```python
from build123d import *
from build123d.topology import SkipClean

# Parameters (mm, degrees)
BOSS_EXTRUDE1_DEPTH                  = 15
SKETCH2_R                            = 12.5
BOSS_EXTRUDE2_DEPTH                  = 22
BOSS_EXTRUDE2_DIRECTION_2_REACH      = 23.768
BOSS_EXTRUDE2_DIRECTION_2_END_RADIUS = 40.5
SKETCH3_R                            = 9.9
BOSS_EXTRUDE3_DEPTH                  = 13
CHAMFER1_SIZE                        = 1
FILLET7_R                            = 3


with BuildPart() as part:
    # Sketch1 → Boss-Extrude1 (new, symmetric)
    with BuildSketch(Plane(origin=(0, 0, 0), x_dir=(1, 0, 0), z_dir=(0, 1, 0))):
        with BuildLine():
            ThreePointArc((2.261526721, 12.825755375), (0, 0), (2.261526721, -12.825755375))
            ThreePointArc((2.261526721, -12.825755375), (1.365018004, -14.748324521), (-0.557551142, -13.851815805))
            ThreePointArc((-0.557551142, -13.851815805), (-3, 0), (-0.557551142, 13.851815805))
            ThreePointArc((-0.557551142, 13.851815805), (1.365018004, 14.748324521), (2.261526721, 12.825755375))
        make_face()
    extrude(amount=BOSS_EXTRUDE1_DEPTH, both=True)

    # Sketch2 → Boss-Extrude2 (add)
    with BuildSketch(Plane.ZY.offset(3)):
        with Locations(Location((0, 0, 0), (0, 0, 180))):
            Circle(SKETCH2_R)
    extrude(amount=BOSS_EXTRUDE2_DEPTH)

    # Boss-Extrude2 direction 2: up to this cylinder (the profile starts outside it)
    with SkipClean():  # the faces are left unmerged after this step: merging them gives an invalid solid
        boss_extrude2_direction_2_end = Plane(origin=(37.5, 0, 0), z_dir=(0, -1, 0)) * Cylinder(BOSS_EXTRUDE2_DIRECTION_2_END_RADIUS, 129.536, mode=Mode.PRIVATE)
        # Sketch2 → Boss-Extrude2 direction 2 (add, up to the surface)
        with BuildSketch(Plane.ZY.offset(3), mode=Mode.PRIVATE) as boss_extrude2_direction_2_sk1:
            with Locations(Location((0, 0, 0), (0, 0, 180))):
                Circle(SKETCH2_R)
        boss_extrude2_direction_2_tool1 = extrude(boss_extrude2_direction_2_sk1.sketch, amount=-BOSS_EXTRUDE2_DIRECTION_2_REACH, mode=Mode.PRIVATE) - boss_extrude2_direction_2_end
        add(boss_extrude2_direction_2_tool1.solids().sort_by_distance((-3, 0, 0))[0])
        add(boss_extrude2_direction_2_tool1.solids().sort_by_distance((-3, 0, 0))[1])

    # Sketch3 → Boss-Extrude3 (add)
    with BuildSketch(Plane.ZY.offset(25)):
        with Locations(Location((0, 0, 0), (0, 0, 180))):
            Circle(SKETCH3_R)
    extrude(amount=BOSS_EXTRUDE3_DEPTH)

    # Chamfer1
    chamfer1_edges = [part.edges().sort_by_distance(p)[0] for p in [
        (-38, 0, 9.9),
    ]]
    chamfer(chamfer1_edges, length=CHAMFER1_SIZE)

    # Fillet7
    fillet7_edges = [part.edges().sort_by_distance(p)[0] for p in [
        (-1.022720569, 0, 12.5),
    ]]
    fillet(fillet7_edges, radius=FILLET7_R)


solid = part.part
```
The model under review builds one solid part; all positions refer to its coordinate system, in mm. A direction names the side the tool comes from. Round coordinates to 2 decimals unless told otherwise and drop trailing zeros. Write each loop counter-clockwise with the first axis right and the second up, starting at its lowest first coordinate (ties: lowest second). Pieces come first, ordered by that corner, then holes. Notation, with made-up numbers: (41.5, 65) - (69.5, 65) arc R18 ccw to (69.5, 86) - close; hole circle Ø7 at (30.5, 27). An arc over 180 degrees is marked (long way). One line per question, with ' | ' between items.
Item 1: For faces 4 (the face through (-1.46, -12.41, -11.06)), 5 (the face through (-1.34, -12.02, 11.48)), 6 (the face through (-1.46, 12.46, -11.06)), 7 (the face through (-13.868, -3.755, -11.923)), 8 (the face through (-0.3, -15, -0.2)), list the 3-axis set-ups (+Z, -Z, +X, -X, +Y, -Y) from which the entire face can be reached by the end or side of a thin tool; tool diameter is ignored.
Resolved:
face 4: -Z, -X, -Y | face 5: +Z, -X, -Y | face 6: -Z, -X, +Y | face 7: -X | face 8: +Z, -Z, +X, -X, -Y
Item 2: Add section A-A, the plane x = -9. Give the boundary of the cut face in (y, z), then the cut area to 3 significant figures.
Resolved:
outline: circle Ø25 at (0, 0) | area: 491 mm2
Item 3: To check wall thickness, follow probe 1 along X at (y, z) = (8, 0.25); probe 2 along Y at (x, z) = (-14, -3.5); probe 3 along Z at (x, y) = (-16, 0.5). State the ranges of each line that lie inside material, in increasing order.
Resolved:
probe 1: x = -38 to 0 | probe 2: y = -12 to 12 | probe 3: z = -12.49 to 12.49
Item 4: Add section B-B, the plane x = -35. Give the boundary of the cut face in (y, z).
Resolved:
outline: circle Ø19.8 at (0, 0)
Item 5: The part is to be moulded in two halves that separate along Z. For faces 1 (the face through (0, 0, 0)), 2 (the face through (-0.3, 15, -0.2)), 3 (the face through (-1.45, 12.07, 11.1)), say which applies: pulls with the +Z half, pulls with the -Z half, needs draft (parallel to the pull), parting line crosses it, or undercut.
Resolved:
face 1: undercut | face 2: needs draft | face 3: pulls with the +Z half
Item 6: For P1, Ø10, axis at x = -11.5, z = 7.5, coming from the +Y side; P2, Ø4, axis at y = -1.5, z = -11, coming from the -X side; P3, Ø8, axis at x = -13, z = -2, coming from the +Y side, all flat-tipped, find the tip position at first contact; note any pin that passes through.
Resolved:
P1: stops at y = 12.25 | P2: stops at x = -37.8 | P3: stops at y = 12.5
